Autodesk Inventor part; units mm, degrees
ref_plane "YZ Plane" through (0, 0, 0) normal (1, 0, 0) x (0, 1, 0)
ref_plane "XZ Plane" through (0, 0, 0) normal (0, 1, 0) x (-1, 0, 0)
ref_plane "XY Plane" through (0, 0, 0) normal (0, 0, 1) x (1, 0, 0)
sketch "Sketch1" plane through (0, 0, 0) normal (0, 1, 0) x (-1, 0, 0)
  line L0 (28.305, -41.33) -> (-28.305, -41.33)
  line L1 (-28.305, -41.33) -> (-28.305, 41.33)
  line L2 (-28.305, 41.33) -> (28.305, 41.33)
  line L3 (28.305, 41.33) -> (28.305, -41.33)
  point P0 (0, 0)
  dimension "d0" = 56.61
  dimension "d1" = 82.66
  dimension "d2" = 41.33
  dimension "d3" = 28.305
extrude "Extrusion1" add sketch "Sketch1" along normal blind 1.7
sketch "Sketch2" plane through (0, 1.7, 0) normal (0, 1, 0) x (1, 0, 0)
  line L0 (28.305, 41.33) -> (-28.305, 41.33)
  line L1 (28.305, -41.33) -> (28.305, 41.33)
  line L2 (25, 20.43) -> (35, 20.43) construction
  line L3 (25, 17.115) -> (35, 17.115)
  line L4 (35, 23.745) -> (25, 23.745)
  arc A0 (25, 23.745) -> (25, 17.115) centre (25, 20.43) ccw
  arc A1 (35, 17.115) -> (35, 23.745) centre (35, 20.43) ccw
  line L5 (0, 0) -> (0, 18.0494) construction
  line L6 (-25, 20.43) -> (-35, 20.43) construction
  line L7 (-25, 17.115) -> (-35, 17.115)
  line L8 (-35, 23.745) -> (-25, 23.745)
  arc A2 (-25, 17.115) -> (-25, 23.745) centre (-25, 20.43) ccw
  arc A3 (-35, 23.745) -> (-35, 17.115) centre (-35, 20.43) ccw
  line L9 (-28.305, -41.33) -> (28.305, -41.33)
  line L10 (0, 0) -> (21.685, 0) construction
  line L11 (25, -20.43) -> (35, -20.43) construction
  line L12 (25, -17.115) -> (35, -17.115)
  line L13 (35, -23.745) -> (25, -23.745)
  arc A4 (25, -17.115) -> (25, -23.745) centre (25, -20.43) ccw
  arc A5 (35, -23.745) -> (35, -17.115) centre (35, -20.43) ccw
  line L14 (-25, -20.43) -> (-35, -20.43) construction
  line L15 (-25, -17.115) -> (-35, -17.115)
  line L16 (-35, -23.745) -> (-25, -23.745)
  arc A6 (-25, -23.745) -> (-25, -17.115) centre (-25, -20.43) ccw
  arc A7 (-35, -17.115) -> (-35, -23.745) centre (-35, -20.43) ccw
  point P0 (30, 20.43)
  point P1 (-30, 20.43)
  point P2 (30, -20.43)
  point P3 (-30, -20.43)
  dimension "d6" = 6.63
  dimension "d8" = 6.62
  dimension "d9" = 10
  dimension "d27" = 40.86
  dimension "d28" = 20.9
  dimension "d29" = 20.43
  dimension "d30" = 20.43
  dimension "d31" = 41.33
  dimension "d32" = 41.33
  dimension "d33" = 20.9
extrude "Extrusion2" cut sketch "Sketch2" against normal through all
sketch "Sketch3" plane through (0, 1.7, 0) normal (0, 1, 0) x (1, 0, 0)
  line L0 (-28.305, 17.115) -> (-28.305, -41.33)
  line L1 (-28.305, -41.33) -> (28.305, -41.33)
  line L2 (-28.305, 41.33) -> (-28.305, 23.745)
  point P0 (0, 0)
  point P1 (-13.995, -27)
  point P2 (14.005, -27)
  point P3 (14.005, 27)
  point P4 (-13.995, 27)
  dimension "d12" = 14.31
  dimension "d13" = 14.33
  dimension "d14" = 28
  dimension "d15" = 28
  dimension "d16" = 54
  dimension "d17" = 14.33
  dimension "d18" = 14.31
  dimension "d19" = 54
hole "Hole1" at (-13.995, 1.7, 27) at (14.005, 1.7, 27) at (14.005, 1.7, -27) at (-13.995, 1.7, -27) direction (0, -1, 0) diameter 3.2 end through all
sketch "Sketch4" plane through (0, 1.7, 0) normal (0, 1, 0) x (1, 0, 0)
  line L0 (-28.305, -41.33) -> (28.305, -41.33)
  line L1 (28.305, 41.33) -> (-28.305, 41.33)
  line L2 (-28.305, 17.115) -> (-28.305, -17.115)
  line L3 (18, -8) -> (-18, -8) construction
  line L4 (-18, -8) -> (-18, 8) construction
  line L5 (-18, 8) -> (18, 8) construction
  line L6 (18, 8) -> (18, -8) construction
  line L7 (18, -8) -> (-18, 8) construction
  line L8 (-18, -8) -> (18, 8) construction
  point P0 (0, 0)
  point P1 (0, 0)
  dimension "d34" = 36
  dimension "d35" = 16
  dimension "d36" = 28.305
  dimension "d37" = 56.61
  dimension "d38" = 82.66
  dimension "d39" = 41.33
hole "Hole2" at (-18, 1.7, -8) at (-18, 1.7, 8) at (18, 1.7, 8) at (18, 1.7, -8) direction (0, -1, 0) diameter 2 end through all
sketch "Sketch5" plane through (0, 1.7, 0) normal (0, 1, 0) x (1, 0, 0)
  line L0 (-28.305, -23.745) -> (-28.305, -41.33)
  line L1 (-28.305, -41.33) -> (28.305, -41.33)
  circle A0 centre (-18.535, -30.07) radius 1
  circle A1 centre (-7.105, -30.07) radius 1
  point P0 (0, 0)
  dimension "d47" = 9.77
  dimension "d48" = 11.26
  dimension "d49" = 21.2
  dimension "d50" = 11.26
  dimension "d51" = 2
  dimension "d52" = 2
  dimension "d53" = 11.43
extrude "Extrusion3" cut sketch "Sketch5" against normal through all
sketch "Sketch6" plane through (0, 1.7, 0) normal (0, 1, 0) x (1, 0, 0)
  line L0 (-28.352, 41.33) -> (28.305, 41.33) construction
  line L1 (28.305, 41.33) -> (28.305, -41.33) construction
  line L2 (28.305, -41.33) -> (-28.352, -41.33) construction
  line L3 (-28.352, -41.33) -> (-28.352, 41.33) construction
  line L4 (28.305, 41.33) -> (-28.305, 41.33)
  line L5 (-28.305, -41.33) -> (28.305, -41.33)
  line L6 (28.305, -17.115) -> (28.305, 17.115)
  point P0 (0, 0)
decal "Decal1"
sketch "Sketch7" plane through (0, 0, 0) normal (0, -1, 0) x (1, 0, 0)
  line L0 (-28.352, 41.33) -> (28.305, 41.33) construction
  line L1 (28.305, 41.33) -> (28.305, -41.33) construction
  line L2 (28.305, -41.33) -> (-28.352, -41.33) construction
  line L3 (-28.352, -41.33) -> (-28.352, 41.33) construction
  line L4 (28.305, 41.33) -> (-28.305, 41.33)
  line L5 (-28.305, -41.33) -> (28.305, -41.33)
  line L6 (28.305, -17.115) -> (28.305, 17.115)
  point P0 (0, 0)
decal "Decal2"
equation "\"d52\" = d51"
properties part number "PCB"
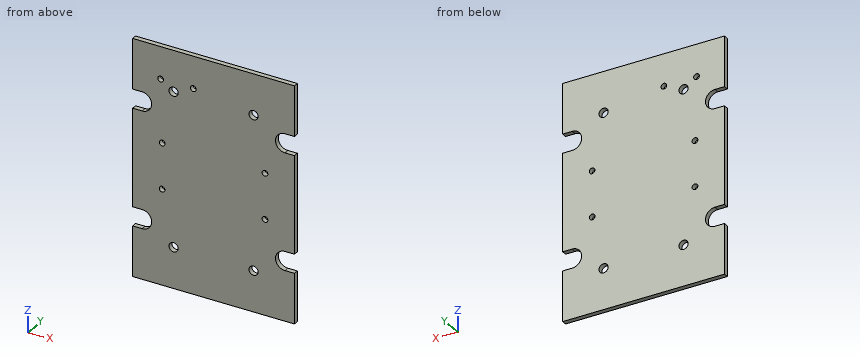
For this review, take the finished solid that the model builds, in its own axes (mm). Give positions to 0.01 mm unless a question says otherwise; leave off trailing zeros. Loops run counter-clockwise (first coordinate to the right, second up) from the corner with the lowest first, then second, coordinate; pieces in that order, holes last. Notation, with made-up numbers: M 77.5,21 L 93.5,21 A27 ccw 93.5,44 Z; hole C 66,-25 d6. An arc over 180 degrees is marked long. One line per item, written item: value. Start each with the question number.
Q1. Add section B-B (z = -8). Give the boundary of the cut face in (x, y) (3 decimals), and give its area (3 significant figures).
Q2. For L1, parallel to Z at x = -14, y = 1; L2, parallel to X at y = 0.5, z = 8 (3 decimals); L3, parallel to X at y = 0.5, z = 30.07 (3 decimals), list the stretches that pass through material, from the lowest coordinate up.
Q3. Add section A-A (x = 18). Give the boundary of the cut face in (y, z).
Q4. Add section C-C (y = 1.25). Count the separate pieces of the cut face and the enclosed holes in it, and give its area (3 significant figures).
Q5. Add section D-D (z = -20.43). Give the boundary of the cut face in (x, y) (3 decimals).
Reply:
1. outline: M -28.305,0 L -19,0 L -19,1.7 L -28.305,1.7 Z; M -17,0 L 17,0 L 17,1.7 L -17,1.7 Z; M 19,0 L 28.305,0 L 28.305,1.7 L 19,1.7 Z
1. area: 89.4 mm²
2. L1: -41.33 to -28.6, -25.4 to 25.4, 28.6 to 41.33
2. L2: -28.305 to -19, -17 to 17, 19 to 28.305
2. L3: -28.305 to -19.535, -17.535 to -8.105, -6.105 to 28.305
3. outline: M 0,-41.33 L 1.7,-41.33 L 1.7,-9 L 0,-9 Z; M 0,-7 L 1.7,-7 L 1.7,7 L 0,7 Z; M 0,9 L 1.7,9 L 1.7,41.33 L 0,41.33 Z
4. separate pieces: 1
4. enclosed holes: 10
4. area: 4,470 mm²
5. outline: M -21.685,0 L 21.685,0 L 21.685,1.7 L -21.685,1.7 Z
